Geometry: final body of the model. Coordinates: model frame, mm. Face numbers are marked on the shaded views. A direction names the side the tool comes from. Coordinates: 2 decimals unless noted, no trailing zeros. Order: outer loops, then holes, each group sorted by start corner. A loop starts at its lowest first (then second) coordinate and runs counter-clockwise, first axis right, second up. Notation, with made-up numbers: (73, 44.25) -> (82, 44.25) arc R20 ccw to (82, 59.25) -> close; hole circle Ø4 at (73, 89). An arc over 180 degrees is marked (long way). Answer in a Markdown table with one row per item. Add a question column.
1) Section query A-A on z = 74. Return the cut outline in (x, y).
2) Ray query, line 1 (Y direction, x = 29.5, z = 53.5); line 2 (X direction, y = 63, z = 122.5); line 3 (Y direction, x = -114.5, z = 119). Return the intervals inside material, ascending. Write a range as from..to.
3) Set-up query: the marked faces 4 and 5. Return all of +Z, -Z, +X, -X, +Y, -Y with unobstructed straight access to the full face (end or side cutting, diameter ignored); none if empty.
4) Section query C-C on x = 170.5. Return the cut outline in (y, z), then the cut area to 3 significant figures.
5) Section query B-B on y = 8. Return the cut outline in (x, z), then the cut area to 3 significant figures.
6) Pull-direction query (Y, two-part tool) for the marked faces 1, 2 and 3; classes: +Y half, -Y half, draft (parallel to the pull), parting line (faces both ways), or undercut.
7) Contact query for flat-ended pins moving along their axis: P1, Ø1, axis at x = -67.5, y = -22.5, coming from the +Z side; P2, Ø6, axis at x = -0.5, z = 136, coming from the -Y side; P3, Ø2.5, axis at x = 9, z = 119, coming from the +Y side. Output: stop coordinate, or through.
Solid Edge part; units mm, degrees
sketch "Sketch1" plane through (0, 0, 0) normal (0, 0, 1) x (1, 0, 0)
  line L0 (-210, 80) -> (-210, -80)
  line L1 (-210, -80) -> (210, -80)
  line L2 (210, -80) -> (210, 80)
  line L3 (210, 80) -> (-210, 80)
extrude "Protrusion1" add sketch "Sketch1" along normal blind 145
shell "Thinwall_2" thickness 15 removed faces 1 at (-144.2, -51.7333, 145)
sketch "Sketch2" plane through (0, -80, 72.5) normal (0, -1, 0) x (1, 0, 0)
  line L0 (-6, 64.5) -> (6, 64.5)
  line L1 (6, 64.5) -> (6, 54.5)
  line L2 (6, 54.5) -> (-6, 54.5)
  line L3 (-6, 54.5) -> (-6, 64.5)
extrude "Cutout1" cut sketch "Sketch2" against normal blind 10
sketch "Sketch3" plane through (0, -80, 72.5) normal (0, -1, 0) x (1, 0, 0)
  line L0 (-6, 67.5) -> (6, 67.5)
  line L1 (6, 67.5) -> (6, 64.5)
  line L2 (6, 64.5) -> (-6, 64.5)
  line L3 (-6, 64.5) -> (-6, 67.5)
extrude "Cutout2" cut sketch "Sketch3" against normal blind 10
sketch "Sketch4" plane through (210, 0, 72.5) normal (1, 0, 0) x (0, 1, 0)
  line L0 (-75, 47.5) -> (-80, 47.5)
  line L1 (-80, 47.5) -> (-80, 44.5)
  line L2 (-80, 44.5) -> (-75, 44.5)
  line L3 (-75, 44.5) -> (-75, 47.5)
  line L4 (75, 49.5) -> (80, 49.5)
  line L5 (80, 49.5) -> (80, 44.5)
  line L6 (80, 44.5) -> (75, 44.5)
  line L7 (75, 44.5) -> (75, 49.5)
extrude "Cutout3" cut sketch "Sketch4" against normal up to next
properties material "ABS Plastic, high impact"
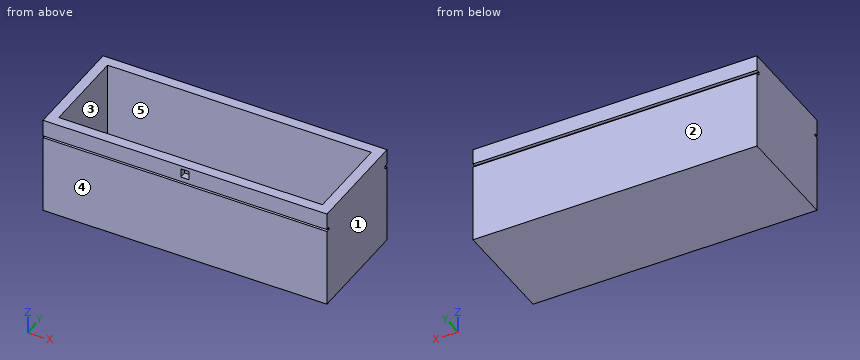
Result:
| question | item | result |
|---|---|---|
| 1 | outline | (-210, -80) -> (210, -80) -> (210, 80) -> (-210, 80) -> close; hole (-195, -65) -> (195, -65) -> (195, 65) -> (-195, 65) -> close |
| 2 | line 1 | -80..-65, 65..80 |
| 2 | line 2 | -210..-195, 195..210 |
| 2 | line 3 | -75..-65, 65..75 |
| 3 | face 4 | +Z, -Z, +X, -X, -Y |
| 3 | face 5 | +Z |
| 4 | outline | (-80, 0) -> (80, 0) -> (80, 117) -> (75, 117) -> (75, 122) -> (80, 122) -> (80, 145) -> (65, 145) -> (65, 15) -> (-65, 15) -> (-65, 145) -> (-80, 145) -> (-80, 120) -> (-75, 120) -> (-75, 117) -> (-80, 117) -> close |
| 4 | area | 6,260 mm2 |
| 5 | outline | (-210, 0) -> (210, 0) -> (210, 145) -> (195, 145) -> (195, 15) -> (-195, 15) -> (-195, 145) -> (-210, 145) -> close |
| 5 | area | 10,200 mm2 |
| 6 | face 1 | draft |
| 6 | face 2 | +Y half |
| 6 | face 3 | undercut |
| 7 | P1 | z = 15 |
| 7 | P2 | y = -70 |
| 7 | P3 | y = 75 |
